Part model, mm, in its own coordinate system. A direction names the side the tool comes from. Coordinates: 2 decimals unless noted, no trailing zeros. Write each loop counter-clockwise with the first axis right and the second up, starting at its lowest first coordinate (ties: lowest second). Pieces come first, ordered by that corner, then holes. Notation, with made-up numbers: (18.25, 1) -> (52.25, 1) arc R13 cw to (52.25, 14) -> close; hole circle Ø7 at (89.25, 37). An arc over 180 degrees is marked (long way). Write item = value, one per line.
from build123d import *

# Parameters (mm, degrees)
SKETCH4_R           = 2
BOSS_EXTRUDE3_DEPTH = 12
SKETCH5_R           = 3
CUT_EXTRUDE1_DEPTH  = 3
FILLET2_R           = 9


with BuildPart() as part:
    # Sketch4 → Boss-Extrude3 (new body)
    with BuildSketch(Plane(origin=(0, 0, 0), x_dir=(1, 0, 0), z_dir=(0, 1, 0))):
        with BuildLine():
            ThreePointArc((-15.743367066, -13.557035328), (-1.346456096, -10.041025711), (13.451962467, -9.240914984))
            ThreePointArc((13.451962467, -9.240914984), (14.223098903, -3.176461435), (15.743367066, 2.744774328))
            ThreePointArc((15.743367066, 2.744774328), (0.886180468, 6.912573541), (-13.040688221, 13.557035328))
            ThreePointArc((-13.040688221, 13.557035328), (-5.710452271, -0.865362874), (-15.743367066, -13.557035328))
        make_face()
        with Locations(Location((-0.236677372, -1.605971843, 0), (0, 0, 270))):
            Circle(SKETCH4_R, mode=Mode.SUBTRACT)
        with Locations(Location((9.704188058, -2.691879069, 0), (0, 0, 270))):
            Circle(SKETCH4_R, mode=Mode.SUBTRACT)
    extrude(amount=BOSS_EXTRUDE3_DEPTH)

    # Sketch5 → Cut-Extrude1 (cut)
    with BuildSketch(Plane(origin=(0, 12, 0), x_dir=(1, 0, 0), z_dir=(0, 1, 0))):
        with Locations(Location((-0.236677372, -1.605971843, 0), (0, 0, 270))):
            Circle(SKETCH5_R)
        with Locations(Location((9.704188058, -2.691879069, 0), (0, 0, 270))):
            Circle(SKETCH5_R)
    extrude(amount=-CUT_EXTRUDE1_DEPTH, mode=Mode.SUBTRACT)

    # Fillet2
    # the kernel refuses this fillet: 9 mm, written as the material it takes off along each edge
    with BuildSketch(Plane(origin=(62.351465844, 12, 12.377564393), x_dir=(-0.9229460384493624, 0, 0.38492935729900885), z_dir=(0.38492935729900885, 0, 0.9229460384493624))) as fillet2_piece_1:
        with BuildLine():
            CenterArc((49 + FILLET2_R, FILLET2_R), FILLET2_R, 180, 90)
            Line((49 + FILLET2_R, 0), (49, 0))
            Line((49, 0), (49, FILLET2_R))
        make_face()
    revolve(axis=Axis((62.351465844, 12, 12.377564393), (0, -1, 0)), revolution_arc=66.924942426, mode=Mode.SUBTRACT)


solid = part.part
Q1. Pin check, flat tips, straight feed: pin 1 (5 mm diameter, centred on y = 8, z = 6.5, fed in from -X); pin 2 (5.5 mm diameter, centred on x = -0.24, z = 1.61, fed in from +Y); pin 3 (5 mm diameter, centred on y = 2.5, z = 7.5, fed in from +X); pin 4 (3.5 mm diameter, centred on x = -0.24, z = 1.61, fed in from -Y). Stop position of each tip, or through.
Model answer:
pin_1 = -9.13
pin_2 = 9
pin_3 = 13.91
pin_4 = through
Q2. Saw through at D-D on z = 1.75. Count the separate pieces of the cut face and the enclosed holes in it, and give its area (3 significant figures).
Model answer:
separate_pieces = 3
enclosed_holes = 0
area = 131 mm²
Q3. Saw through at B-B on y = 2. Give the cut face in (x, z).
Model answer:
outline = (-15.74, 13.56) arc R15 cw to (-13.04, -13.56) arc R90 cw to (15.74, -2.74) arc R49 cw to (13.45, 9.24) arc R80 cw to start; hole circle Ø4 at (-0.24, 1.61); hole circle Ø4 at (9.7, 2.69)
Q4. Mould opens along X. For faces 1 (the face through (-2.062, 10.521, -0.775)), 2 (the face through (14.2, 1.5, 3.3)), 3 (the face through (3, 0, 3)), 4 (the face through (-1, 9, 4)) say: released by +X, released by -X, zero draft, split by the parting line, or undercut.
Model answer:
face_1 = undercut
face_2 = released by +X
face_3 = zero draft
face_4 = undercut
Q5. Probe line 1 (X direction, y = 7.5, z = 2); line 2 (Z direction, x = -11, y = 9.25); line 3 (Z direction, x = 4.5, y = 4.75). List the from-to ranges inside material, lowest first. Write a range as from..to.
Model answer:
line_1 = -5.87..-2.2, 1.72..7.83, 11.58..13.23
line_2 = -12.39..-12.12, 10.87..12.08
line_3 = -5.64..9.4
Q6. Saw through at A-A on x = -7.5. Give the cut face in (y, z), and give its area (3 significant figures).
Model answer:
outline = (0, -10.56) -> (12, -10.56) -> (12, -7.86) -> (0, -7.86) -> close; (0, 6.62) -> (12, 6.62) -> (12, 11.2) -> (0, 11.2) -> close
area = 87.3 mm²
Q7. Saw through at C-C on y = 10.5. Give the cut face in (x, z), and give its area (3 significant figures).
Model answer:
outline = (-15.74, 13.56) arc R15 cw to (-13.04, -13.56) arc R90 cw to (11.79, -3.59) arc R53.03 cw to (10.81, -0.1) arc R3 cw (long way) to (9.75, 5.69) arc R53.03 cw to (9.42, 9.19) arc R80 cw to start; hole circle Ø6 at (-0.24, 1.61)
area = 250 mm²
Q8. Which spindle directions (+Z, -Z, +X, -X, +Y, -Y) get a long thin tool onto all of the face, cutting with end or side? Do faces 5 (the face through (11.687, 4.437, 2.432)), 6 (the face through (8.9, 9, 0.6)), 7 (the face through (-1.55, 5.92, 10.07)). Say none if no direction does.
Model answer:
face_5 = +Y, -Y
face_6 = +Y
face_7 = +Z, +Y, -Y
